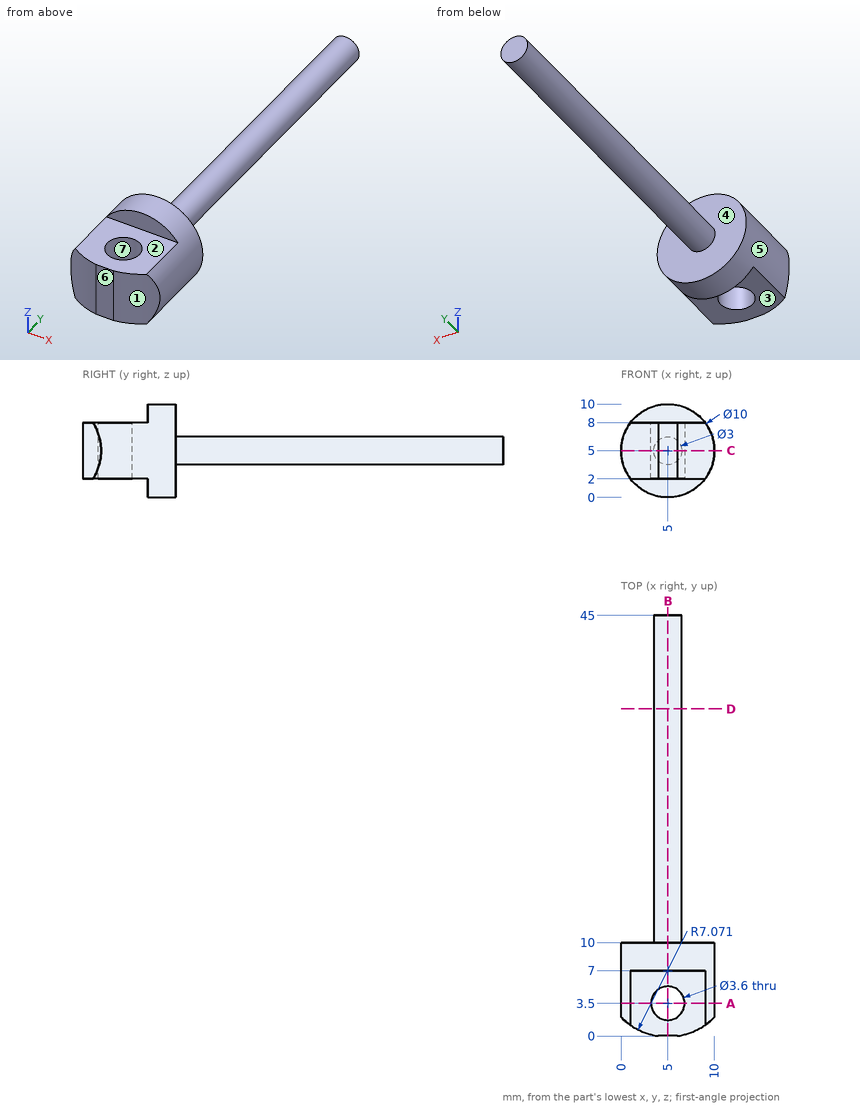
Study the drawing (mm; zero at the part's minimum x, y, z) and answer. A direction names the side the tool comes from. Give positions to 0.01 mm unless a question says otherwise; leave off trailing zeros. Write each loop counter-clockwise with the first axis right and the second up, starting at its lowest first coordinate (ties: lowest second). Pieces come first, ordered by that corner, then holes.
Item 1: Which of the six approach directions +Z, -Z, +X, -X, +Y, -Y give full straight-line access (tool end or side, diameter ignored) to the marked faces 1, 2, 3 and 4?
Item 2: Section A-A, the plane y = 3.5 is taken. Write down the section's boundary in (x, z).
Item 3: Section D-D, the plane y = 35 is taken. Write down the section's boundary in (x, z), plus the area to 3 significant figures.
Item 4: Section B-B, the plane x = 5 is taken. Write down the section's boundary in (y, z).
Item 5: Flat-ended cylindrical pins translate along their axes: P1, Ø2, axis at x = 3.5, y = 3, coming from the -Z side; P2, Ø3, axis at x = 6, z = 7, coming from the +Y side; P3, Ø6, axis at y = 9.5, z = 1.5, coming from the -X side (3 decimals); P4, Ø2, axis at x = 4, y = 35, coming from the -Z side. Find the tip coordinate at first contact, or state that the pin passes through.
Item 6: Determine the mould class of the marked faces 5, 6 and 7 for opening direction X: released by +X, released by -X, zero draft, split by the parting line, or undercut.
Item 7: Section C-C, the plane z = 5 is taken. Write down the section's boundary in (x, y).
Item 8: Find the intervals of material crossed by line 1 along Y through (x, z) = (5, 6.1); line 2 along Y through (x, z) = (5, 6.6); line 3 along Z through (x, y) = (4.75, 9.5), in increasing order.
Completed:
1. face 1: +Z, -Z, +X, -Y
1. face 2: +Z, +X, -X, -Y
1. face 3: -Z, +X, -X, -Y
1. face 4: +Y
2. outline: (1, 2) - (3.2, 2) - (3.2, 8) - (1, 8) arc R5 ccw to start; (6.8, 2) - (9, 2) arc R5 ccw to (9, 8) - (6.8, 8) - close
3. outline: circle Ø3 at (5, 5)
3. area: 7.07 mm2
4. outline: (0, 2) - (1.7, 2) - (1.7, 8) - (0, 8) - close; (5.3, 2) - (7, 2) - (7, 0) - (10, 0) - (10, 3.5) - (45, 3.5) - (45, 6.5) - (10, 6.5) - (10, 10) - (7, 10) - (7, 8) - (5.3, 8) - close
5. P1: stops at z = 2
5. P2: stops at y = 45
5. P3: stops at x = 0.025
5. P4: stops at z = 3.5
6. face 5: split by the parting line
6. face 6: zero draft
6. face 7: undercut
7. outline: (0, 2) arc R7.07 ccw to (4, 0) - (6, 0) arc R7.07 ccw to (10, 2) - (10, 10) - (6.5, 10) - (6.5, 45) - (3.5, 45) - (3.5, 10) - (0, 10) - close; hole circle Ø3.6 at (5, 3.5)
8. line 1: y = 0 to 1.7, 5.3 to 45
8. line 2: y = 0 to 1.7, 5.3 to 10
8. line 3: z = 0.01 to 9.99
